```python
from build123d import *

# Parameters (mm, degrees)
SKETCH1_W           = 50
SKETCH1_H           = 50
SKETCH1_R           = 1.5
BOSS_EXTRUDE1_DEPTH = 2


with BuildPart() as part:
    # Sketch1 → Boss-Extrude1 (new body)
    with BuildSketch(Plane(origin=(0, 0, 0), x_dir=(1, 0, 0), z_dir=(0, 1, 0))):
        Rectangle(SKETCH1_W, SKETCH1_H)
        with Locations(Location((8.5, -8.5, 0), (0, 0, 270))):
            Circle(SKETCH1_R, mode=Mode.SUBTRACT)
        with Locations(Location((-8.5, -8.5, 0), (0, 0, 270))):
            Circle(SKETCH1_R, mode=Mode.SUBTRACT)
        with BuildLine():
            Line((-10.002005601, 4.390529846), (-10.002005601, 12.719094592))
            ThreePointArc((-10.002005601, 12.719094592), (-8.502005601, 14.219094592), (-7.002005601, 12.719094592))
            Line((-7.002005601, 12.719094592), (-7.002005601, 4.390529846))
            ThreePointArc((-7.002005601, 4.390529846), (-8.502005601, 2.890529846), (-10.002005601, 4.390529846))
        make_face(mode=Mode.SUBTRACT)
        with BuildLine():
            Line((7, 4.335717627), (7, 12.664282373))
            ThreePointArc((7, 12.664282373), (8.5, 14.164282373), (10, 12.664282373))
            Line((10, 12.664282373), (10, 4.335717627))
            ThreePointArc((10, 4.335717627), (8.5, 2.835717627), (7, 4.335717627))
        make_face(mode=Mode.SUBTRACT)
        with BuildLine():
            Line((-1.870832872, -1.293852114), (-1.870832872, 7.034712631))
            ThreePointArc((-1.870832872, 7.034712631), (-0.370832872, 8.534712631), (1.129167128, 7.034712631))
            Line((1.129167128, 7.034712631), (1.129167128, -1.293852114))
            ThreePointArc((1.129167128, -1.293852114), (-0.370832872, -2.793852114), (-1.870832872, -1.293852114))
        make_face(mode=Mode.SUBTRACT)
    extrude(amount=BOSS_EXTRUDE1_DEPTH)


solid = part.part
```
For this review, take the finished solid that the model builds, in its own axes (mm). A direction names the side the tool comes from. Coordinates: 2 decimals unless noted, no trailing zeros. Order: outer loops, then holes, each group sorted by start corner. A loop starts at its lowest first (then second) coordinate and runs counter-clockwise, first axis right, second up. Notation, with made-up numbers: (4, 76.25) - (38, 76.25) arc R35 cw to (38, 108.25) - close; hole circle Ø3 at (-0.5, 74). An arc over 180 degrees is marked (long way). Answer as a JSON object with one key per item and string values. Group by question number.
1. The part is to be moulded in two halves that separate along X. For faces 1 (the flat face through (0, 2, 5)), 2 (the flat face through (-10.002, 1, -8)), 3 (the flat face through (25, 1, 0)), say which applies: pulls with the +X half, pulls with the -X half, needs draft (parallel to the pull), parting line crosses it, or undercut.
2. We need section D-D on z = 8.5. State the section outline as (x, y) points.
3. We need section B-B on x = 8.5. State the section outline as (y, z) points.
4. For faces 4 (the flat face through (7, 1, -8)), 5 (the flat face through (0, 1, -25)), list the 3-axis set-ups (+Z, -Z, +X, -X, +Y, -Y) from which the entire face can be reached by the end or side of a thin tool; tool diameter is ignored.
5. We need section A-A on z = -2. State the section outline as (x, y) points, then the cut area to 3 significant figures.
6. For probe 1 along X at (y, z) = (1.1, 8.5); probe 2 along X at (y, z) = (0.4, 1); probe 3 along X at (y, z) = (0.6, -4), list the stretches that pass through material, from the lowest coordinate up.
7. We need section C-C on y = 1.05. State the section outline as (x, z) points.
Final values:
{
 "1": {"face 1": "needs draft", "face 2": "undercut", "face 3": "pulls with the +X half"},
 "2": {"outline": "(-25, 0) - (-10, 0) - (-10, 2) - (-25, 2) - close; (-7, 0) - (7, 0) - (7, 2) - (-7, 2) - close; (10, 0) - (25, 0) - (25, 2) - (10, 2) - close"},
 "3": {"outline": "(0, -25) - (2, -25) - (2, -14.16) - (0, -14.16) - close; (0, -2.84) - (2, -2.84) - (2, 7) - (0, 7) - close; (0, 10) - (2, 10) - (2, 25) - (0, 25) - close"},
 "4": {"face 4": "+Y, -Y", "face 5": "-Z, +X, -X, +Y, -Y"},
 "5": {"outline": "(-25, 0) - (-1.87, 0) - (-1.87, 2) - (-25, 2) - close; (1.13, 0) - (25, 0) - (25, 2) - (1.13, 2) - close", "area": "94.0 mm²"},
 "6": {"probe 1": "-25 to -10, -7 to 7, 10 to 25", "probe 2": "-25 to -1.87, 1.13 to 25", "probe 3": "-25 to -9.95, -7.05 to -1.87, 1.13 to 7.04, 9.96 to 25"},
 "7": {"outline": "(-25, -25) - (25, -25) - (25, 25) - (-25, 25) - close; hole (-10, -12.72) arc R1.5 ccw to (-7, -12.72) - (-7, -4.39) arc R1.5 ccw to (-10, -4.39) - close; hole circle Ø3 at (-8.5, 8.5); hole (-1.87, -7.03) arc R1.5 ccw to (1.13, -7.03) - (1.13, 1.29) arc R1.5 ccw to (-1.87, 1.29) - close; hole (7, -12.66) arc R1.5 ccw to (10, -12.66) - (10, -4.34) arc R1.5 ccw to (7, -4.34) - close; hole circle Ø3 at (8.5, 8.5)"}
}
